from build123d import *

# Parameters (mm, degrees)
SKETCH_1_W      = 20
SKETCH_1_H      = 20
SKETCH_1_R      = 1.5
EXTRUDE_1_DEPTH = 3
CHAMFER_1_SIZE  = 5
EXTRUDE_2_DEPTH = 7


with BuildPart() as part:
    # 草图1 → 凸台-拉伸1 (new body)
    with BuildSketch(Plane(origin=(0, 0, 0), x_dir=(1, 0, 0), z_dir=(0, 1, 0))):
        Rectangle(SKETCH_1_W, SKETCH_1_H)
        with Locations(Location((0, 0, 0), (0, 0, 270))):
            Circle(SKETCH_1_R, mode=Mode.SUBTRACT)
    extrude(amount=EXTRUDE_1_DEPTH)

    # 倒角1
    chamfer_1_edges = [part.edges().sort_by_distance(p)[0] for p in [
        (-10, 1.5, 10),
        (10, 1.5, -10),
    ]]
    chamfer(chamfer_1_edges, length=CHAMFER_1_SIZE)

    # 草图2 → 凸台-拉伸2 (add)
    with BuildSketch(Plane(origin=(0, 3, 0), x_dir=(1, 0, 0), z_dir=(0, 1, 0))):
        Polygon((10, -10), (10, 5), (5, 10), (-10, 10), (-10, -5), (-5, -10), align=None)
        Polygon((-7, 7), (-7, -3.757359313), (-3.757359313, -7), (7, -7), (7, 3.757359313), (3.757359313, 7), align=None, mode=Mode.SUBTRACT)
    extrude(amount=EXTRUDE_2_DEPTH)


solid = part.part
Input: part model. Units: mm. Frame: model coordinates. A direction names the side the tool comes from. Round coordinates to 2 decimals unless told otherwise and drop trailing zeros. Order: outer loops, then holes, each group sorted by start corner. A loop starts at its lowest first (then second) coordinate and runs counter-clockwise, first axis right, second up. Notation, with made-up numbers: (30, -11) - (86, -11) arc R20 cw to (86, 28) - close; hole circle Ø5 at (-31.5, 44.25). An arc over 180 degrees is marked (long way). Use a Markdown table: item, result.
1. Access query for faces 5 (the face through (7, 6, 2)), 6 (the face through (10, 5, 3)). Directions: +Z, -Z, +X, -X, +Y, -Y. A direction counts if a zero-diameter tool reaches every point of the face in a straight line with its end or side. Return the directions, or none.
Evaluation:
| item | result |
|---|---|
| face 5 | +Y |
| face 6 | +Z, -Z, +X, +Y, -Y |
2. Material intervals for probe 1 along Z at (x, y) = (1.25, 5.5); probe 2 along X at (y, z) = (0.7, 0), sorted ascending.
Evaluation:
| item | result |
|---|---|
| probe 1 | -10 to -7, 7 to 10 |
| probe 2 | -10 to -1.5, 1.5 to 10 |
3. Section C-C on x = 0. Return the cut outline in (y, z).
Evaluation:
| item | result |
|---|---|
| outline | (0, -10) - (10, -10) - (10, -7) - (3, -7) - (3, -1.5) - (0, -1.5) - close; (0, 1.5) - (3, 1.5) - (3, 7) - (10, 7) - (10, 10) - (0, 10) - close |
4. First-contact query: pin 1 (1.8 mm diameter, centred on x = 0, z = 0, fed in from +Y). Flat tip, straight axial feed; report the tip coordinate or a pass-through.
Evaluation:
| item | result |
|---|---|
| pin 1 | through |
5. Section A-A on y = 8.25. Return the cut outline in (x, z), then the cut area to 3 significant figures.
Evaluation:
| item | result |
|---|---|
| outline | (-10, -10) - (5, -10) - (10, -5) - (10, 10) - (-5, 10) - (-10, 5) - close; hole (-7, -7) - (3.76, -7) - (7, -3.76) - (7, 7) - (-3.76, 7) - (-7, 3.76) - close |
| area | 190 mm^2 |
6. Section B-B on z = 0. Return the cut outline in (x, y).
Evaluation:
| item | result |
|---|---|
| outline | (-10, 0) - (-1.5, 0) - (-1.5, 3) - (-7, 3) - (-7, 10) - (-10, 10) - close; (1.5, 0) - (10, 0) - (10, 10) - (7, 10) - (7, 3) - (1.5, 3) - close |
7. Mould query, pull axis Z, two halves, no side actions, for faces 1 (the face through (4, 10, -7)), 2 (the face through (-7, 6, -2)), 3 (the face through (8, 5, -7)), 4 (the face through (-8, 5, 7)). Classes: +Z half, -Z half, draft (parallel to the pull), parting line (faces both ways), or undercut.
Evaluation:
| item | result |
|---|---|
| face 1 | draft |
| face 2 | undercut |
| face 3 | -Z half |
| face 4 | +Z half |
8. Section D-D on x = 8. Return the cut outline in (y, z).
Evaluation:
| item | result |
|---|---|
| outline | (0, -7) - (10, -7) - (10, 10) - (0, 10) - close |
